from build123d import *

# Parameters (mm, degrees)
F0_R     = 12
F0_R_2   = 6.5
F0_R_3   = 3.75
F0_R_4   = 1.75
F1_DEPTH = 1.5
F2_DEPTH = 3.5
F3_DEPTH = 0.6
F4_SIZE  = 1
F5_SIZE  = 1.2


with BuildPart() as f1:
    # F0 (on Top) → F1 (new body)
    with BuildSketch(Plane.XY):
        Circle(F0_R)
        Circle(F0_R_2, mode=Mode.SUBTRACT)
        Circle(F0_R_2)
        Circle(F0_R_3, mode=Mode.SUBTRACT)
        Circle(F0_R_3)
        Circle(F0_R_4, mode=Mode.SUBTRACT)
    extrude(amount=-F1_DEPTH)

    # F0 (on Top) → F2 (join)
    with BuildSketch(Plane.XY):
        Circle(F0_R_3)
        Circle(F0_R_4, mode=Mode.SUBTRACT)
    extrude(amount=F2_DEPTH)

    # F0 (on Top) → F3 (join)
    with BuildSketch(Plane.XY):
        Circle(F0_R_2)
        Circle(F0_R_3, mode=Mode.SUBTRACT)
    extrude(amount=F3_DEPTH)

    # F4
    f4_edges = [f1.edges().sort_by_distance(p)[0] for p in [
        (-12, 0, -1.5),
    ]]
    chamfer(f4_edges, length=F4_SIZE)

    # F5
    f5_edges = [f1.edges().sort_by_distance(p)[0] for p in [
        (-1.75, 0, -1.5),
    ]]
    chamfer(f5_edges, length=F5_SIZE)


solid = f1.part
Here's how the part is built. I have some questions about the finished solid (model axes, mm). A direction names the side the tool comes from. Round coordinates to 2 decimals unless told otherwise and drop trailing zeros. Loops run counter-clockwise (first coordinate to the right, second up) from the corner with the lowest first, then second, coordinate; pieces in that order, holes last. Notation, with made-up numbers: (23.25, 6) - (78.25, 6) arc R19 cw to (78.25, 20) - close; hole circle Ø1 at (-23, -16.5). An arc over 180 degrees is marked (long way). One line per question, with ' | ' between items. Start each with the question number.
Q1. Will these pins go through, and if not, where does the flat tip stop? pin 1 (1 mm diameter, centred on y = -5.5, z = -1, fed in from -X); pin 2 (4 mm diameter, centred on x = 1, y = -8, fed in from +Z).
Q2. I want a section at D-D (z = -0.9). Write out the boundary of the cut face in (x, y), then the cut area to 3 significant figures.
Q3. Please list where these lines run through material, in increasing order: line 1 (Y direction, x = 0, z = 1.4); line 2 (Y direction, x = 0, z = 0.5); line 3 (Z direction, x = -9.75, y = 5). Write a range as [from, to].
Q4. I want a section at A-A (y = 0). Write out the boundary of the cut face in (x, z), then the cut area to 3 significant figures.
Q5. For faces 4 (the cylindrical face through (-3.746, 0.165, 2.03)), 5 (the flat face through (2.3, -2.3, -1.5)), which set-ups out of +Z, -Z, +X, -X, +Y, -Y let a thin tool reach every point of the face, with its end or its side?
Q6. We'd pull the mould along X, two halves only. Please class faces 1 (the cylindrical face through (1.617, -0.67, 1.573)), 2 (the cylindrical face through (-5.158, -3.955, 0.296)), 3 (the flat face through (2, -1, 3.5)): +X half, -X half, draft (parallel to the pull), parting line (faces both ways), or undercut.
Q7. I want a section at C-C (z = 1.45). Write out the boundary of the cut face in (x, y), then the cut area to 3 significant figures.
Response values:
1) pin 1: stops at x = -10.72 | pin 2: stops at z = 0.6
2) outline: circle Ø23.2 at (0, 0); hole circle Ø4.7 at (0, 0) | area: 405 mm²
3) line 1: y = [-3.75, -1.75], [1.75, 3.75] | line 2: y = [-6.5, -1.75], [1.75, 6.5] | line 3: z = [-1.5, 0]
4) outline: (-12, -0.5) - (-11, -1.5) - (-2.95, -1.5) - (-1.75, -0.3) - (-1.75, 3.5) - (-3.75, 3.5) - (-3.75, 0.6) - (-6.5, 0.6) - (-6.5, 0) - (-12, 0) - close; (1.75, -0.3) - (2.95, -1.5) - (11, -1.5) - (12, -0.5) - (12, 0) - (6.5, 0) - (6.5, 0.6) - (3.75, 0.6) - (3.75, 3.5) - (1.75, 3.5) - close | area: 45.6 mm²
5) face 4: +Z | face 5: -Z, +X, -X, +Y, -Y
6) face 1: undercut | face 2: parting line | face 3: draft
7) outline: circle Ø7.5 at (0, 0); hole circle Ø3.5 at (0, 0) | area: 34.6 mm²
